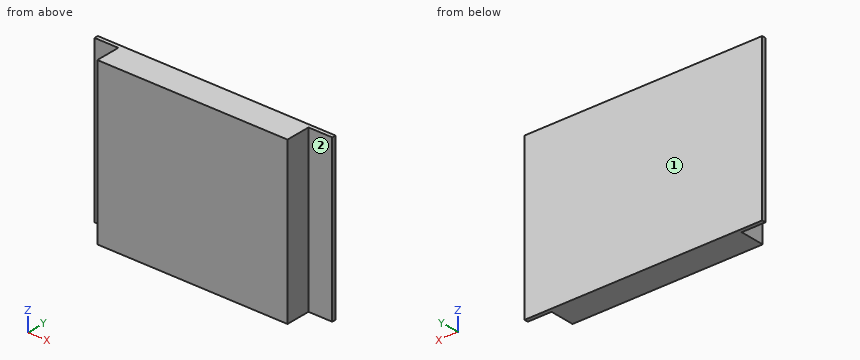
```python
from build123d import *

# Parameters (mm, degrees)
SKETCH1_W           = 200
SKETCH1_H           = 30
SKETCH1_W_2         = 25
SKETCH1_H_2         = 4
BOSS_EXTRUDE1_DEPTH = 85


with BuildPart() as part:
    # Sketch1 → Boss-Extrude1 (new, symmetric)
    with BuildSketch(Plane.XY):
        Rectangle(SKETCH1_W, SKETCH1_H)
        with Locations((-112.5, 13)):
            Rectangle(SKETCH1_W_2, SKETCH1_H_2)
        with Locations((112.5, 13)):
            Rectangle(SKETCH1_W_2, SKETCH1_H_2)
    extrude(amount=BOSS_EXTRUDE1_DEPTH, both=True)


solid = part.part
```
Here's how the part is built. I have some questions about the finished solid (model axes, mm). Face numbers are marked on the shaded views. A direction names the side the tool comes from. Round coordinates to 2 decimals unless told otherwise and drop trailing zeros. Write each loop counter-clockwise with the first axis right and the second up, starting at its lowest first coordinate (ties: lowest second). Pieces come first, ordered by that corner, then holes. Notation, with made-up numbers: M 23.5,17.5 L 35.5,17.5 A22 ccw 35.5,44.5 Z; hole C 70.25,71 d2. An arc over 180 degrees is marked long. Answer as CSV lines item,"result". Start each with the question number.
1. Suppose I cut it at A-A on z = 60. Write out the boundary of the cut face in (x, y).
2. I need wall thicknesses on probe 1 along X at (y, z) = (2, 59.5); probe 2 along Y at (x, z) = (111, 60.5). Which ranges of each line are inside material? Lowest first, please.
3. Suppose I cut it at B-B on y = -12. Write out the boundary of the cut face in (x, z), then the cut area to 3 significant figures.
4. On a 3-axis mill with a long thin cutter (end or side, diameter ignored), from which of +Z, -Z, +X, -X, +Y, -Y can I reach the whole of each face in a straight line? I mean the marked faces 1 and 2. Say none if no direction works.
5. I'm going to push flat-ended pins straight in: pin 1 Ø12.5 at (x, z) = (-114, -28) entering from -Y; pin 2 Ø8 at (y, z) = (2, 10) entering from +X. Where does each tip first touch, or does it pass through?
Check result:
1,outline,"M -125,11 L -100,11 L -100,-15 L 100,-15 L 100,11 L 125,11 L 125,15 L -125,15 Z"
2,probe 1,"x = -100 to 100"
2,probe 2,"y = 11 to 15"
3,outline,"M -100,-85 L 100,-85 L 100,85 L -100,85 Z"
3,area,"34,000 mm2"
4,face 1,"+Z, -Z, +X, -X, +Y"
4,face 2,"+Z, -Z, +X, -Y"
5,pin 1,"stops at y = 11"
5,pin 2,"stops at x = 100"
